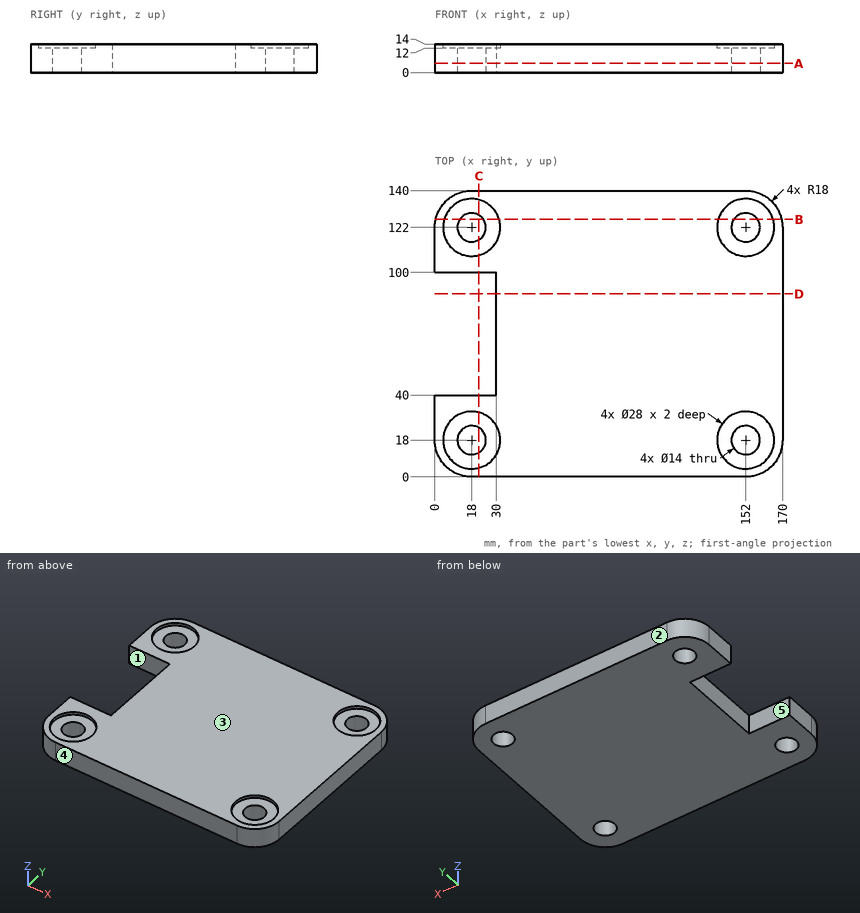
Geometry check sheet. Reference: drawing and pictorial views, mm from the part's lowest x, y, z. A direction names the side the tool comes from. Round coordinates to 2 decimals unless told otherwise and drop trailing zeros. Loops run counter-clockwise (first coordinate to the right, second up) from the corner with the lowest first, then second, coordinate; pieces in that order, holes last. Notation, with made-up numbers: (51, 74) -> (103, 74) arc R16 cw to (103, 81) -> close; hole circle Ø10 at (16.25, -16). An arc over 180 degrees is marked (long way). Answer as a JSON object with one key per item and string values. Group by question number.
Item 1: Thickness scan on line 1 along Y through (x, z) = (152, 13.55); line 2 along Y through (x, z) = (15.5, 4.75); line 3 along X through (y, z) = (88, 6.25). Record the ranges inside material, lowest first.
Item 2: Depth check by flat-ended pin: pin 1 Ø4 at (x, z) = (12.5, 4.5) entering from +Y; pin 2 Ø1 at (y, z) = (78, 1.5) entering from -X; pin 3 Ø22.5 at (x, y) = (20, 18) entering from +Z. Enter the tip coordinate at first touch or a pass-through.
Item 3: Cross-section at C-C, the plane x = 21.5. Record the cut outline in (y, z).
Item 4: Release check for a two-part mould opening along Y. For the marked faces 3, 4 and 5 record: pulls with the +Y half, pulls with the -Y half, needs draft (parallel to the pull), parting line crosses it, or undercut.
Item 5: Cross-section at A-A, the plane z = 4.5. Record the cut outline in (x, y), plus the area to 3 significant figures.
Item 6: Cross-section at B-B, the plane y = 126. Record the cut outline in (x, z).
Item 7: Set-up check for the marked faces 1 and 2: record each of +Z, -Z, +X, -X, +Y, -Y from which the full face is reachable in a straight line by a thin tool's end or side.
Item 8: Cross-section at D-D, the plane y = 89.5. Record the cut outline in (x, z).
Determined:
{
 "1": {"line 1": "y = 0 to 4, 32 to 108, 136 to 140", "line 2": "y = 0.17 to 11.46, 24.54 to 40, 100 to 115.46, 128.54 to 139.83", "line 3": "x = 30 to 170"},
 "2": {"pin 1": "stops at y = 139.66", "pin 2": "stops at x = 30", "pin 3": "stops at z = 12"},
 "3": {"outline": "(0, 0) -> (11.94, 0) -> (11.94, 12) -> (4.44, 12) -> (4.44, 14) -> (0, 14) -> close; (24.06, 0) -> (40, 0) -> (40, 14) -> (31.56, 14) -> (31.56, 12) -> (24.06, 12) -> close; (100, 0) -> (115.94, 0) -> (115.94, 12) -> (108.44, 12) -> (108.44, 14) -> (100, 14) -> close; (128.06, 0) -> (140, 0) -> (140, 14) -> (135.56, 14) -> (135.56, 12) -> (128.06, 12) -> close"},
 "4": {"face 3": "needs draft", "face 4": "pulls with the -Y half", "face 5": "undercut"},
 "5": {"outline": "(0, 18) arc R18 ccw to (18, 0) -> (152, 0) arc R18 ccw to (170, 18) -> (170, 122) arc R18 ccw to (152, 140) -> (18, 140) arc R18 ccw to (0, 122) -> (0, 100) -> (30, 100) -> (30, 40) -> (0, 40) -> close; hole circle Ø14 at (18, 18); hole circle Ø14 at (18, 122); hole circle Ø14 at (152, 18); hole circle Ø14 at (152, 122)", "area": "21,100 mm²"},
 "6": {"outline": "(0.45, 0) -> (12.26, 0) -> (12.26, 12) -> (4.58, 12) -> (4.58, 14) -> (0.45, 14) -> close; (23.74, 0) -> (146.26, 0) -> (146.26, 12) -> (138.58, 12) -> (138.58, 14) -> (31.42, 14) -> (31.42, 12) -> (23.74, 12) -> close; (157.74, 0) -> (169.55, 0) -> (169.55, 14) -> (165.42, 14) -> (165.42, 12) -> (157.74, 12) -> close"},
 "7": {"face 1": "+Z, -Z, -X", "face 2": "+Z, -Z, +X, -X, +Y"},
 "8": {"outline": "(30, 0) -> (170, 0) -> (170, 14) -> (30, 14) -> close"}
}
